Read the model definition and answer for the solid it produces. Units are mm, in the model's axes. Face numbers are marked on the shaded views. A direction names the side the tool comes from. Coordinates: 2 decimals unless noted, no trailing zeros. Write each loop counter-clockwise with the first axis right and the second up, starting at its lowest first coordinate (ties: lowest second). Pieces come first, ordered by that corner, then holes.
(1) The mould has two halves that part along Y. Classify the marked faces 4, 5 and 6: +Y half, -Y half, draft (parallel to the pull), parting line (faces both ways), or undercut.
(2) Section A-A on x = 6 is taken. Write down the section's boundary in (y, z), then the cut area to 3 significant figures.
(3) Find the intervals of material crossed by probe 1 along Y at (x, z) = (-35, 69); probe 2 along Z at (x, y) = (-23, 21); probe 3 along Z at (x, y) = (2, 37), in increasing order.
(4) Given pin 1 (1.5 mm diameter, centred on y = 89, z = -69, fed in from +X); pin 2 (9 mm diameter, centred on x = 5.5, z = 83.5, fed in from -Y), each flat-ended and moving along its own axis, determine where each tip first touches the part or whether it passes through.
(5) Section B-B on z = 50 is taken. Write down the section's boundary in (x, y), then the cut area to 3 significant figures.
(6) Section D-D on x = 32.5 is taken. Write down the section's boundary in (y, z), then the cut area to 3 significant figures.
(7) Which of the six approach directions +Z, -Z, +X, -X, +Y, -Y give full straight-line access (tool end or side, diameter ignored) to the marked faces 1, 2 and 3?
(8) Section C-C on y = 49 is taken. Write down the section's boundary in (x, z).
Autodesk Inventor part; units mm, degrees
ref_plane "YZ Plane" through (0, 0, 0) normal (1, 0, 0) x (0, 1, 0)
ref_plane "XZ Plane" through (0, 0, 0) normal (0, 1, 0) x (-1, 0, 0)
ref_plane "XY Plane" through (0, 0, 0) normal (0, 0, 1) x (1, 0, 0)
sketch "Sketch1" plane through (0, 0, 0) normal (0, 1, 0) x (-1, 0, 0)
  line L0 (45, 90) -> (-45, 90)
  line L1 (-45, 90) -> (-45, -90)
  line L2 (-45, -90) -> (45, -90)
  line L3 (45, -90) -> (45, 90)
  point P0 (0, 0)
  dimension "d0" = 180
  dimension "d1" = 90
  dimension "d2" = 45
  dimension "d3" = 90
extrude "Extrusion1" add sketch "Sketch1" along normal blind 140
sketch "Sketch2" plane through (45, 0, 90) normal (1, 0, 0) x (0, 0, -1)
  line L0 (3, 137) -> (177, 137)
  line L1 (177, 137) -> (177, 3)
  line L2 (177, 3) -> (3, 3)
  line L3 (3, 3) -> (3, 137)
  line L4 (0, 140) -> (180, 140)
  line L5 (0, 0) -> (0, 140)
  point P0 (90, 0)
  dimension "d6" = 3
  dimension "d7" = 3
  dimension "d8" = 174
  dimension "d9" = 134
extrude "Extrusion2" cut sketch "Sketch2" against normal blind 87
sketch "Sketch3" plane through (-45, 0, 90) normal (0, 0, 1) x (1, 0, 0)
  line L0 (90, 0) -> (0, 0)
  line L1 (32.5, 40) -> (57.5, 40)
  line L2 (57.5, 40) -> (57.5, 0)
  line L3 (57.5, 0) -> (32.5, 0)
  line L4 (32.5, 0) -> (32.5, 40)
  line L5 (90, 0) -> (90, 140)
  point P0 (45, 0)
  point P1 (57.5, 20)
  point P2 (32.5, 20)
  dimension "d12" = 25
  dimension "d13" = 32.5
  dimension "d14" = 40
sketch "Sketch4" plane through (-45, 0, 90) normal (0, 0, 1) x (1, 0, 0)
  line L0 (90, 0) -> (0, 0)
  line L1 (30.5, 41.9359) -> (59.5, 41.9359)
  line L2 (59.5, 41.9359) -> (59.5, 0)
  line L3 (59.5, 0) -> (30.5, 0)
  line L4 (30.5, 0) -> (30.5, 41.9359)
  line L5 (90, 0) -> (90, 140)
  point P0 (45, 0)
  dimension "d15" = 29
  dimension "d16" = 30.5
extrude "Extrusion3" add sketch "Sketch4" against normal blind 20
extrude "Extrusion4" cut sketch "Sketch3" against normal blind 18
properties part number "Self_balancing_robot"
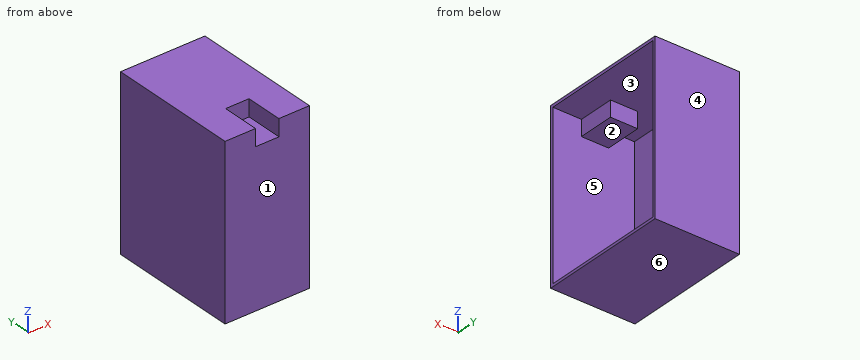
Response:
1. face 4: +Y half
1. face 5: undercut
1. face 6: draft
2. outline: (0, -90) - (140, -90) - (140, 90) - (40, 90) - (40, 72) - (0, 72) - close; hole (3, -87) - (137, -87) - (137, 87) - (41.94, 87) - (41.94, 70) - (3, 70) - close
2. area: 1,830 mm2
3. probe 1: y = 0 to 3, 137 to 140
3. probe 2: z = -90 to -87, 87 to 90
3. probe 3: z = -90 to -87, 70 to 72
4. pin 1: stops at x = -42
4. pin 2: stops at y = 40
5. outline: (-45, 0) - (45, 0) - (45, 3) - (-42, 3) - (-42, 137) - (45, 137) - (45, 140) - (-45, 140) - close
5. area: 942 mm2
6. outline: (0, -90) - (140, -90) - (140, 90) - (0, 90) - close; hole (3, -87) - (137, -87) - (137, 87) - (3, 87) - close
6. area: 1,880 mm2
7. face 1: +Z, -Z, +X, -X, -Y
7. face 2: +X
7. face 3: none
8. outline: (-45, -90) - (45, -90) - (45, -87) - (-42, -87) - (-42, 87) - (45, 87) - (45, 90) - (-45, 90) - close
